Build history of the part. All positions in model axes, mm. Face numbers are marked on the shaded views. A direction names the side the tool comes from. Give positions to 0.01 mm unless a question says otherwise; leave off trailing zeros. Loops run counter-clockwise (first coordinate to the right, second up) from the corner with the lowest first, then second, coordinate; pieces in that order, holes last. Notation, with made-up numbers: (41, -21) -> (45, -21) arc R22 cw to (45, -4) -> close; hole circle Ø2 at (37, 11). An arc over 180 degrees is marked (long way). Answer as a JSON object with one key per item and string values. Group by question number.
Q1. Wall check: probe 1 along X at (y, z) = (3.7, 12.5); probe 2 along Y at (x, z) = (-0.9, 15); probe 3 along Y at (x, z) = (-1.5, 5.5). Give the ranges that are in metal, low to high. Write a range as from..to.
Q2. Band-saw the part on D-D, the plane x = 0.5. Write the cut outline in (y, z).
Q3. Tool access for the marked faces 1, 2 and 3: list every direction of +Z, -Z, +X, -X, +Y, -Y with a clear straight run to the whole face (end or side of a thin tool).
Q4. Two-plate mould, pull along X, no slides. Class the marked faces 4, 5 and 6: pulls with the +X half, pulls with the -X half, needs draft (parallel to the pull), parting line crosses it, or undercut.
Q5. Band-saw the part on A-A, the plane z = 11. Write the cut outline in (x, y).
Q6. Band-saw the part on C-C, the plane y = 3.35. Write the cut outline in (x, z).
Q7. Band-saw the part on B-B, the plane x = -0.4. Write the cut outline in (y, z).
Q8. Drop flat-ended pins along their axis: pin 1 (0.8 mm diameter, centred on x = -1.5, y = 1, fed in from +Z) (3 decimals); pin 2 (1.7 mm diameter, centred on y = 3.5, z = -1, fed in from +X); pin 3 (3 mm diameter, centred on x = -1, z = 14.5, fed in from -Y); pin 4 (3 mm diameter, centred on x = 0, z = 0, fed in from -Y). Give the stop position or say it passes through.
Autodesk Inventor part; units mm, degrees
ref_plane "YZ Plane" through (0, 0, 0) normal (1, 0, 0) x (0, 1, 0)
ref_plane "XZ Plane" through (0, 0, 0) normal (0, 1, 0) x (-1, 0, 0)
ref_plane "XY Plane" through (0, 0, 0) normal (0, 0, 1) x (1, 0, 0)
sketch "スケッチ1" plane through (0, 0, 0) normal (0, 1, 0) x (-1, 0, 0)
  circle A0 centre (0, 0) radius 1.15
  circle A1 centre (0, 0) radius 2
  circle A2 centre (0, 0) radius 2.9
  line L0 (2, 0) -> (-2, 0)
  line L1 (-2, 0) -> (-2, -2.9)
  line L2 (-2, -2.9) -> (2, -2.9)
  line L3 (2, -2.9) -> (2, 0)
  line L4 (0, 0) -> (0, 2.9)
  line L5 (0, 0) -> (2.9, 0)
  line L6 (2.9, 0) -> (2.9, 10)
  line L7 (2.9, 10) -> (0, 10)
  line L8 (0, 10) -> (0, 0)
  point P0 (0, 2)
  point P1 (-2, -2.1)
  point P2 (2, -2.1)
  dimension "d1" = 4
  dimension "d2" = 5.8
  dimension "d0" = 2.3
  dimension "d3" = 10
extrude "押し出し1" add sketch "スケッチ1" along normal blind 3.7 contours A1 L1 A2 L4
extrude "押し出し2" add sketch "スケッチ1" along normal blind 4.8 contours L5 A2 L3 | A1 L4 A2 L5 | A2 L8 L7 L6
sketch "スケッチ2" plane through (0, 4.8, 0) normal (0, 1, 0) x (1, 0, 0)
  circle A0 centre (0, 0) radius 1.15
  circle A1 centre (0, 0) radius 2.0044
  circle A2 centre (0, 0) radius 2.9
  line L0 (2, 2.1) -> (2, 0)
  line L1 (2, 0) -> (-2.0044, 0)
  line L2 (-2.0044, 0) -> (-2.0044, 2.9)
  line L3 (-2.0044, 2.9) -> (2, 2.9)
  line L4 (2, 2.9) -> (2, 0)
  line L5 (0, -10) -> (0, -2)
  line L6 (-2.9, 0) -> (0, 0)
  line L7 (0, 0) -> (0, -10)
  line L8 (0, -10) -> (-2.9, -10)
  line L9 (-2.9, -10) -> (-2.9, 0)
  point P0 (0, -2.9)
  dimension "d8" = 2.3
extrude "押し出し3" add sketch "スケッチ2" along normal blind 0.9 contours L1 L0 A1 L5 L7 A0 | A0 L1 A1 L0 | A0 L7 L5 A1 L1 | L2 A2 L0 A1 | L6 A2 L2 | A1 L5 A2 L6 | L0 A2 L5 A1 | A2 L5 L8 L9
sketch "スケッチ3" plane through (-2.9, 0, 10) normal (0, 0, 1) x (1, 0, 0)
  line L0 (2.9, 0) -> (1.4, 0)
  line L1 (1.4, 0) -> (1.4, 1)
  line L2 (1.4, 1) -> (2.9, 1)
  line L3 (2.9, 1) -> (2.9, 0)
  dimension "d11" = 1.5
  dimension "d12" = 1
hole "穴1" at (-1.5, 1, 10) direction (0, 0, -1) diameter 1 depth 10
sketch "スケッチ4" plane through (-2.9, 0, 10) normal (0, 0, 1) x (1, 0, 0)
  line L0 (0, 0) -> (0, 5.7)
  line L1 (0, 5.7) -> (4, 5.7)
  line L2 (4, 5.7) -> (4, 1.7)
  line L3 (4, 1.7) -> (0, 1.7)
  line L4 (0, 1.7) -> (0, 5.7)
  point P0 (2.9, 0)
  dimension "d20" = 4
  dimension "d21" = 4
extrude "押し出し4" add sketch "スケッチ4" along normal blind 10 and the other way blind 3
fillet "フィレット1" radius 2 1 edges at (1.1, 3.7, 7)
sketch "スケッチ5" plane through (-2.9, 0, 20) normal (0, 0, 1) x (1, 0, 0)
  line L0 (5.8, 5.7) -> (0, 5.7)
  line L1 (0, 5.7) -> (2, 5.7)
  line L2 (2, 5.7) -> (2, 3.7)
  line L3 (2, 3.7) -> (0, 3.7)
  line L4 (0, 3.7) -> (0, 5.7)
  point P0 (2.9, 0)
  point P1 (2.9, 5.7)
  dimension "d27" = 2
  dimension "d28" = 2
hole "穴2" at (-0.9, 3.7, 20) direction (0, 0, -1) diameter 2.3 depth 10
properties part number "srod1.4left"
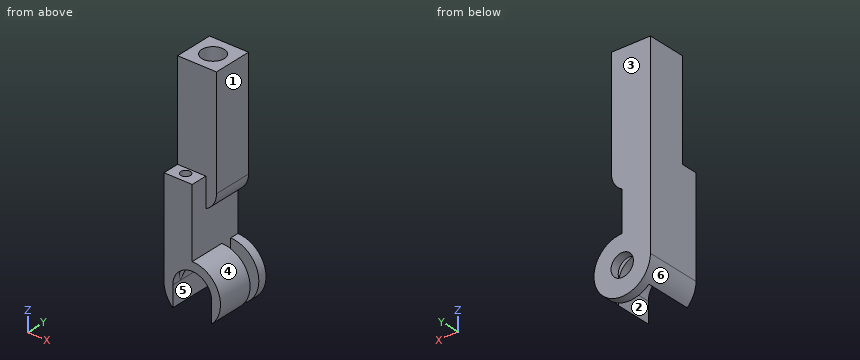
Worked answers:
{
 "1": {"probe 1": "-2.9..-2.05, 0.25..1.1", "probe 2": "1.7..2.55, 4.85..5.7", "probe 3": "0..0.5, 1.5..5.7"},
 "2": {"outline": "(0, 1.94) -> (3.7, 1.94) -> (3.7, 2.86) -> (0, 2.86) -> close; (1.7, 7.36) -> (5.7, 7.36) -> (5.7, 20) -> (1.7, 20) -> close; (4.8, -2.86) -> (5.7, -2.86) -> (5.7, -1.04) -> (4.8, -1.04) -> close; (4.8, 1.04) -> (5.7, 1.04) -> (5.7, 2.86) -> (4.8, 2.86) -> close"},
 "3": {"face 1": "+Z, +X, +Y, -Y", "face 2": "-Z, -Y", "face 3": "+Z, -Z, +X, -X, +Y"},
 "4": {"face 4": "pulls with the +X half", "face 5": "undercut", "face 6": "parting line crosses it"},
 "5": {"outline": "(-2.9, 1.7) -> (1.1, 1.7) -> (1.1, 5.7) -> (-2.9, 5.7) -> close; hole circle Ø2.3 at (-0.9, 3.7)"},
 "6": {"outline": "(-2.9, 0) arc R2.9 ccw to (-2, -2.1) -> (-2, 0) arc R2 cw to (2, 0) -> (2, -2.1) arc R2.9 ccw to (0, 2.9) -> (0, 7) arc R2 ccw to (1.1, 8.79) -> (1.1, 20) -> (0.2, 20) -> (0.2, 10) -> (-2, 10) -> (-2, 20) -> (-2.9, 20) -> close"},
 "7": {"outline": "(0, 1.96) -> (4.8, 1.96) -> (4.8, 1.08) -> (5.7, 1.08) -> (5.7, 20) -> (4.74, 20) -> (4.74, 10) -> (2.66, 10) -> (2.66, 20) -> (1.7, 20) -> (1.7, 10) -> (0, 10) -> close; (4.8, -2.87) -> (5.7, -2.87) -> (5.7, -1.08) -> (4.8, -1.08) -> close"},
 "8": {"pin 1": "through", "pin 2": "x = 2.9", "pin 3": "y = 1.7", "pin 4": "y = 4.8"}
}
